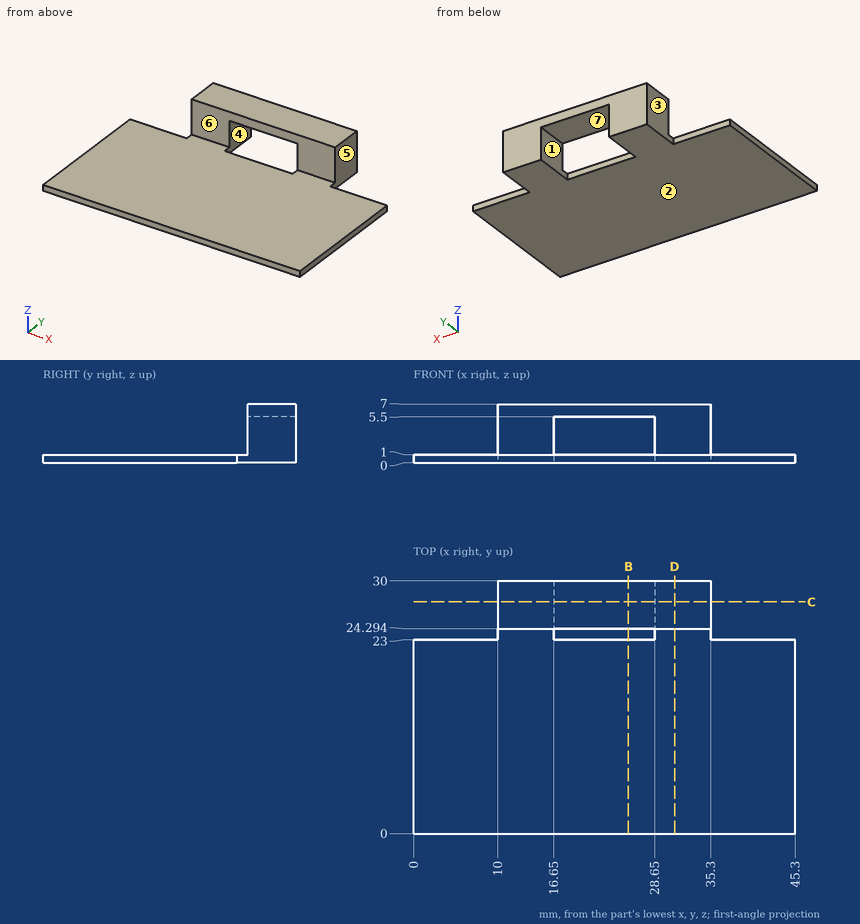
The figure shows three views and two pictorial views of one solid part (mm, origin at its lowest corner). Answer the questions. A direction names the side the tool comes from. Round coordinates to 2 decimals unless told otherwise and drop trailing zeros. Loops run counter-clockwise (first coordinate to the right, second up) from the corner with the lowest first, then second, coordinate; pieces in that order, holes last. Notation, with made-up numbers: M 17,46 L 65,46 A8 ccw 65,54 Z; hole C 82,-16.75 d10. An arc over 180 degrees is marked long. Write each question's results on one line, items separated by ' | '. Start each with the question number.
1) Determine the mould class of the marked faces 1, 2 and 3 for opening direction X: pulls with the +X half, pulls with the -X half, needs draft (parallel to the pull), parting line crosses it, or undercut.
2) Straight lines are drawn through the part: probe 1 along X at (y, z) = (24.5, 0.75); probe 2 along Z at (x, y) = (18.5, 24.5); probe 3 along Z at (x, y) = (13, 3.25). For each, find the intervals that lie inside material, in ascending order.
3) Find section D-D on x = 31. Write down the section's boundary in (y, z) (1 decimal).
4) Find section B-B on x = 25.5. Write down the section's boundary in (y, z) (1 decimal).
5) Each of these flat-tipped pins is pushed along its axis until it touches: pin 1 (0.8 mm diameter, centred on x = 3, z = 0.5, fed in from +Y); pin 2 (1.7 mm diameter, centred on x = 21.5, y = 26.5, fed in from -Z); pin 3 (1 mm diameter, centred on x = 12.5, z = 3, fed in from -Y). Where does it stop, or does it pass through?
6) Which of the six approach directions +Z, -Z, +X, -X, +Y, -Y give full straight-line access (tool end or side, diameter ignored) to the marked faces 4, 5, 6 and 7?
7) Find section C-C on y = 27.5. Write down the section's boundary in (x, z).
Final values:
1) face 1: undercut | face 2: needs draft | face 3: pulls with the -X half
2) probe 1: 10 to 16.65, 28.65 to 35.3 | probe 2: 5.5 to 7 | probe 3: 0 to 1
3) outline: M 0,0 L 30,0 L 30,7 L 24.3,7 L 24.3,1 L 0,1 Z
4) outline: M 0,0 L 23,0 L 23,1 L 0,1 Z; M 24.3,5.5 L 30,5.5 L 30,7 L 24.3,7 Z
5) pin 1: y = 23 | pin 2: z = 5.5 | pin 3: y = 24.29
6) face 4: -Z, +Y | face 5: +Z, -Z, +X, +Y | face 6: +Z, +X, -X, -Y | face 7: -Z, +Y, -Y
7) outline: M 10,0 L 16.65,0 L 16.65,5.5 L 28.65,5.5 L 28.65,0 L 35.3,0 L 35.3,7 L 10,7 Z
